Build history of the part. All positions in model axes, mm. Give positions to 0.01 mm unless a question says otherwise; leave off trailing zeros. Order: outer loops, then holes, each group sorted by start corner. A loop starts at its lowest first (then second) coordinate and runs counter-clockwise, first axis right, second up. Notation, with made-up numbers: (-16, 69) -> (17, 69) arc R24 cw to (17, 101) -> close; hole circle Ø2 at (9, -10). An arc over 180 degrees is marked (long way). One line per question, with ' | ' between items. Start each with the question number.
(1) Drill centre lines: L1, parallel to X at y = -0.5, z = 7.5; L2, parallel to X at y = 1.75, z = 3; L3, parallel to Y at x = 0, z = 26.15. Where is each one in solid material? Low to high. Write a range as from..to.
(2) Pull direction X, two halves, no side cores. Call faces 1 (the face through (-0.867, -3.905, 12.675)), 2 (the face through (-2, 2, 0)), 3 (the face through (-0.27, 1.22, 26.02)): +X half, -X half, draft (parallel to the pull), parting line (faces both ways), or undercut.
(3) Cut at A-A (x = 0). Give the cut face in (y, z).
(4) Pin check, flat tip, straight feed: pin 1 Ø1 at (x, y) = (-1, -0.5) entering from -Z. Stop position of the tip, or through.
(5) Cut at C-C (z = 8). Give the cut face in (x, y).
from build123d import *

# Parameters (mm, degrees)
F0_W     = 4
F0_H     = 25
F2_R     = 2.5
F3_DEPTH = 25
F4_R     = 1.25
F5_DEPTH = 25


with BuildPart() as f1:
    # F0 (on Front) → F1 (revolve)
    with BuildSketch(Plane.XZ):
        with Locations((2, 12.5)):
            Rectangle(F0_W, F0_H)
        Polygon((0, 28), (0, 25), (4, 25), align=None)
    revolve(axis=Axis((0, 0, 12.5), (0, 0, 1)))

    # F2 (on face) → F3 (cut)
    with BuildSketch(Plane(origin=(0, 0, 0), x_dir=(1, 0, 0), z_dir=(0, 0, -1))):
        Circle(F2_R)
    extrude(amount=-F3_DEPTH, mode=Mode.SUBTRACT)

    # F4 (on face) → F5 (cut)
    with BuildSketch(Plane(origin=(0, 0, 25), x_dir=(1, 0, 0), z_dir=(0, 0, -1))):
        Circle(F4_R)
    extrude(amount=-F5_DEPTH, mode=Mode.SUBTRACT)


solid = f1.part
Result set:
1) L1: x = -3.97..-2.45, 2.45..3.97 | L2: x = -3.6..-1.79, 1.79..3.6 | L3: y = -2.47..-1.25, 1.25..2.47
2) face 1: parting line | face 2: draft | face 3: undercut
3) outline: (-4, 0) -> (-2.5, 0) -> (-2.5, 25) -> (-1.25, 25) -> (-1.25, 27.06) -> (-4, 25) -> close; (1.25, 25) -> (2.5, 25) -> (2.5, 0) -> (4, 0) -> (4, 25) -> (1.25, 27.06) -> close
4) pin 1: stops at z = 25
5) outline: circle Ø8 at (0, 0); hole circle Ø5 at (0, 0)
